Design review of the part built by this model. Coordinates are the model's own, in mm. A direction names the side the tool comes from. Coordinates: 2 decimals unless noted, no trailing zeros. Loops run counter-clockwise (first coordinate to the right, second up) from the corner with the lowest first, then second, coordinate; pieces in that order, holes last.
Autodesk Inventor part; units mm, degrees
ref_plane "Arbeitsebene2" through (0, 360, 0) normal (0, 1, 0) x (1, 0, 0)
ref_plane "YZ Plane" through (0, 0, 0) normal (1, 0, 0) x (0, 1, 0)
ref_plane "XZ Plane" through (0, 0, 0) normal (0, 1, 0) x (-1, 0, 0)
sketch "Skizze1" plane through (0, 0, 0) normal (0, 1, 0) x (-1, 0, 0)
  line L0 (599, 100) -> (-599, 100)
  line L1 (-599, 100) -> (-599, -100)
  line L2 (-599, -100) -> (599, -100)
  line L3 (599, -100) -> (599, 100)
  line L4 (838.6, 0) -> (-838.6, 0) construction
  line L5 (0, -140) -> (0, 140) construction
  point P0 (0, 0)
  dimension "d0" = 1198
  dimension "d1" = 200
extrude "Extrusion1" add sketch "Skizze1" along normal blind 420
shell "Wandung1" thickness 5 removed faces 1 at (199.6667, 0, -33.3333)
sketch "Skizze2" plane through (-599, 0, 100) normal (0, 0, 1) x (1, 0, 0)
  line L0 (0, 0) -> (1198, 0) construction
  line L1 (1198, 0) -> (1098, 0)
  line L2 (1098, 0) -> (1098, 130)
  line L3 (1098, 130) -> (1098, 360)
  point P0 (599, 0)
  dimension "d9" = 100
  dimension "d10" = 130
  dimension "d11" = 230
hole "Bohrung1" at (499, 360, 100) direction (0, 0, -1) diameter 30 depth 20 tip angle 118
ref_plane "Arbeitsebene1" through (0, 310.83, 0) normal (0, 1, 0) x (1, 0, 0)
sketch "Skizze3" plane through (0, 310.83, 0) normal (0, 1, 0) x (1, 0, 0)
  line L0 (599, 100) -> (-599, 100) construction
  line L1 (599, -100) -> (599, 100) construction
  line L2 (-599, -100) -> (599, -100) construction
  line L3 (-599, 100) -> (-599, -100) construction
  line L4 (599, -100) -> (499, -100)
  line L5 (499, -100) -> (511.5, -100)
  line L6 (499, -100) -> (486.5, -100)
  line L7 (-599, 100) -> (599, 100)
  line L8 (599, 100) -> (599, -100)
  line L9 (599, -100) -> (-599, -100)
  line L10 (-599, -100) -> (-599, 100)
  line L11 (599, 0) -> (86.8278, 0)
  line L12 (499, -100) -> (499, 0)
  line L13 (499, 0) -> (499, 100)
  line L14 (499, 0) -> (536.585, 0)
  line L15 (499, 0) -> (463.415, 0)
  line L16 (499, 0) -> (464.19, 0)
  line L17 (499, 0) -> (499, 36.585)
  line L18 (499, 36.585) -> (535.585, 36.585)
  line L19 (535.585, 36.585) -> (441.933, 36.585)
  line L20 (441.933, 36.585) -> (441.933, -36.585)
  line L21 (441.933, -36.585) -> (535.585, -36.585)
  line L22 (535.585, -36.585) -> (535.585, -71.395)
  line L23 (535.585, -71.395) -> (441.933, -71.395)
  line L24 (441.933, -71.395) -> (407.123, -71.395)
  line L25 (407.123, -71.395) -> (407.123, 36.585)
  line L26 (407.123, 36.585) -> (407.123, 71.395)
  line L27 (407.123, 71.395) -> (535.585, 71.395)
  line L28 (535.585, 71.395) -> (535.585, 36.585)
  point P0 (0, 0)
  dimension "d20" = 100
  dimension "d21" = 12.5
  dimension "d22" = 12.5
  dimension "d33" = 36.585
  dimension "d34" = 36.585
  dimension "d35" = 93.652
  dimension "d36" = 73.17
  dimension "d37" = 93.652
  dimension "d38" = 34.81
  dimension "d39" = 34.81
  dimension "d40" = 34.81
extrude "Extrusion2" add sketch "Skizze3" against normal blind 20
sketch "Skizze6" plane through (-599, 0, 100) normal (0, 0, 1) x (1, 0, 0)
  circle A0 centre (1098, 360) radius 15 construction
  line L0 (5, 310.83) -> (1193, 310.83) construction
  arc A1 (1113, 360) -> (1083, 360) centre (1098, 360) ccw
  line L1 (1083, 360) -> (1083, 310.83)
  line L2 (1113, 360) -> (1113, 310.83)
  circle A2 centre (1098, 360) radius 15
  point P0 (599, 0)
  dimension "d25" = 30
extrude "Extrusion3" add sketch "Skizze3" along normal blind 85 contours L23 L24 L25 L11 L20 L21 L12 | L12 L21 L22 L23 | L27 L28 L18 L13 | L13 L19 L20 L11 L25 L26 L27
ref_plane "Arbeitsebene2" through (0, 360, 0) normal (0, 1, 0) x (1, 0, 0)
sketch "Skizze7" plane through (0, 0, 0) normal (0, 0, 1) x (1, 0, 0)
  circle A0 centre (499, 360) radius 15 construction
  circle A1 centre (499, 360) radius 32
  circle A2 centre (499, 360) radius 32
  point P0 (0, 0)
  dimension "d44" = 64
extrude "Extrusion4" cut sketch "Skizze7" along normal mid plane 107.17
sketch "Skizze8" plane through (0, 420, 0) normal (0, 1, 0) x (1, 0, 0)
  line L0 (-599, 100) -> (599, 100)
  line L1 (599, 100) -> (599, -100)
  line L2 (599, -100) -> (-599, -100)
  line L3 (-599, -100) -> (-599, 100)
  point P0 (0, 0)
extrude "Extrusion5" cut sketch "Skizze8" against normal blind 5
hole "Bohrung2" at (499, 360, 100) direction (0, 0, -1) diameter 20 depth 500 tip angle 118
sketch "Skizze9" plane through (441.933, 310.83, -36.585) normal (1, 0, 0) x (0, 0, -1)
  line L0 (0, 0) -> (0, 85) construction
  line L1 (-73.17, 85) -> (0, 85) construction
  line L2 (-73.17, 0) -> (-73.17, 85) construction
  line L3 (-73.17, 85) -> (0, 85)
  line L4 (-73.17, 85) -> (-73.17, 0)
  line L5 (0, 0) -> (-73.17, 0)
  line L6 (-107.98, 0) -> (34.81, 0) construction
  line L7 (0, 0) -> (0, 85)
  line L8 (-36.585, 0) -> (-36.585, 49.17)
  circle A0 centre (-36.585, 49.17) radius 32
  circle A1 centre (-36.585, 49.17) radius 17.5
  point P0 (-36.585, -310.83)
  dimension "d56" = 49.17
  dimension "d58" = 64
  dimension "d61" = 35
extrude "Extrusion6" cut sketch "Skizze9" against normal blind 5 contours A1 | A0
extrude "Extrusion7" cut sketch "Skizze9" against normal blind 50 contours A1
sketch "Skizze10" plane through (0, 310.83, 0) normal (0, 1, 0) x (1, 0, 0)
  line L0 (-600.9138, 0) -> (-300.0038, 0)
  circle A0 centre (-300.0038, 0) radius 17.5
  line L1 (-300.0038, 0) -> (-206.3518, 0)
  line L2 (-262.3958, 0) -> (-262.3958, 70)
  line L3 (-262.3958, 70) -> (-232.3958, 70)
  line L4 (-232.3958, 70) -> (-232.3958, -70)
  line L5 (-232.3958, -70) -> (-262.3958, -70)
  line L6 (-262.3958, -70) -> (-262.3958, 0)
  line L7 (-300.0038, 0) -> (-263.4188, 0)
  line L8 (-300.0038, 0) -> (-262.3958, 0)
  point P0 (0, 0)
  dimension "d64" = 300.91
  dimension "d72" = 35
  dimension "d74" = 93.652
  dimension "d75" = 70
  dimension "d76" = 30
  dimension "d77" = 140
  dimension "d86" = 36.585
  dimension "d87" = 37.608
hole "Bohrung3" at (-300.0038, 310.83, 0) direction (0, -1, 0) diameter 64 depth 500 tip angle 118
extrude "Extrusion8" add sketch "Skizze10" along normal blind 104.17 contours L2 L3 L4 L1 | L1 L4 L5 L6
sketch "Skizze11" plane through (-262.3958, 310.83, -70) normal (-1, 0, 0) x (0, 0, 1)
  line L0 (-70, 49.17) -> (210, 49.17) construction
  circle A0 centre (70, 49.17) radius 17.5 construction
  circle A1 centre (70, 49.17) radius 32
  circle A2 centre (70, 49.17) radius 17.75
  point P0 (70, -310.83)
  dimension "d80" = 64
  dimension "d83" = 35.5
extrude "Extrusion9" cut sketch "Skizze11" against normal blind 12 contours A1 | A2
extrude "Extrusion10" cut sketch "Skizze11" against normal blind 40 contours A2
sketch "Skizze12" plane through (0, 310.83, 0) normal (0, 1, 0) x (1, 0, 0)
  circle A0 centre (-300.0038, 0) radius 32 construction
  circle A1 centre (-300.0038, 0) radius 40
  circle A2 centre (-300.0038, 0) radius 32
  point P0 (0, 0)
  dimension "d88" = 80
extrude "Extrusion11" add sketch "Skizze12" against normal blind 4
sketch "Skizze13" plane through (0, 0, 0) normal (0, -1, 0) x (1, 0, 0)
  circle A0 centre (-300.0038, 0) radius 32 construction
  circle A1 centre (-300.0038, 0) radius 12.5
  line L0 (-268.0493, -31.9545) -> (-331.9583, 31.9545) construction
  line L1 (-331.9583, -31.9545) -> (-268.0493, 31.9545) construction
  line L2 (-594, 95) -> (594, 95)
  line L3 (594, 95) -> (594, -95)
  line L4 (594, -95) -> (-594, -95)
  line L5 (-594, -95) -> (-594, 95)
  point P0 (0, 0)
  dimension "d101" = 25
extrude "Extrusion12" add sketch "Skizze13" against normal blind 10
sketch "Skizze14" plane through (599, 0, -100) normal (0, 0, -1) x (-1, 0, 0)
  circle A0 centre (100, 360) radius 10 construction
  circle A1 centre (100, 360) radius 15
  point P0 (599, 0)
  dimension "d104" = 30
hole "Bohrung4" at (499, 360, -100) direction (0, 0, 1) diameter 30 depth 20 tip angle 118
sketch "Skizze16" plane through (-232.3958, 310.83, 70) normal (1, 0, 0) x (0, 0, -1)
  circle A0 centre (70, 49.17) radius 17.75 construction
  circle A1 centre (70, 49.17) radius 23.5
  point P0 (70, -310.83)
  dimension "d112" = 47
extrude "Extrusion13" cut sketch "Skizze16" against normal blind 6.4
sketch "Skizze17" plane through (407.123, 310.83, 71.395) normal (-1, 0, 0) x (0, 0, 1)
  circle A0 centre (-71.395, 49.17) radius 17.5 construction
  circle A1 centre (-71.395, 49.17) radius 23.5
  point P0 (-71.395, -310.83)
  dimension "d115" = 47
extrude "Extrusion14" cut sketch "Skizze17" against normal blind 6.4
sketch "Skizze18" plane through (407.123, 310.83, 71.395) normal (0, 0, 1) x (1, 0, 0)
  circle A0 centre (91.877, 49.17) radius 10 construction
  circle A1 centre (91.877, 49.17) radius 16
  point P0 (-407.123, -310.83)
  dimension "d118" = 32
extrude "Extrusion15" cut sketch "Skizze18" against normal blind 7
sketch "Skizze19" plane through (535.585, 310.83, -71.395) normal (0, 0, -1) x (-1, 0, 0)
  circle A0 centre (36.585, 49.17) radius 16 construction
  circle A1 centre (36.585, 49.17) radius 16
  point P0 (535.585, -310.83)
  dimension "d121" = 32
extrude "Extrusion16" cut sketch "Skizze19" against normal blind 7
sketch "Skizze20" plane through (0, 310.83, 0) normal (0, 1, 0) x (1, 0, 0)
  circle A0 centre (-300.0038, 0) radius 32 construction
  circle A1 centre (-300.0038, 0) radius 40
  point P0 (0, 0)
  dimension "d124" = 80
extrude "Extrusion17" cut sketch "Skizze20" against normal blind 12
sketch "Skizze21" plane through (599, 0, -100) normal (0, 0, -1) x (-1, 0, 0)
  circle A0 centre (100, 360) radius 15 construction
  line L0 (1198, 415) -> (0, 415) construction
  line L1 (0, 0) -> (0, 415) construction
  line L2 (0, 0) -> (1198, 0) construction
  line L3 (1198, 0) -> (1198, 415) construction
  point P0 (599, 0)
sketch "Skizze22" plane through (0, 0, 0) normal (0, -1, 0) x (1, 0, 0)
  circle A0 centre (-356.8903, 42.7877) radius 5.0941 construction
  circle A1 centre (-298.864, 3.8435) radius 17.5 construction
  circle A2 centre (-298.864, 3.8435) radius 17.5 construction
  point P0 (0, 0)
  point P1 (-236.8903, 42.7877)
  point P2 (-236.8903, -47.2123)
  point P3 (-356.8903, -47.2123)
  point P4 (-236.8903, 42.7877)
  point P5 (-236.8903, -47.2123)
  point P6 (-356.8903, -47.2123)
hole "Bohrung5" at (-356.8903, 0, 42.7877) at (-236.8903, 0, 42.7877) at (-236.8903, 0, -47.2123) at (-356.8903, 0, -47.2123) direction (0, 1, 0) diameter 9.3762 depth 29.3 tip angle 118
sketch "Skizze23" plane through (0, 415, 0) normal (0, 1, 0) x (1, 0, 0)
  line L0 (-599, 100) -> (599, 100)
  line L1 (599, 100) -> (599, -100)
  line L2 (599, -100) -> (-599, -100)
  line L3 (-599, -100) -> (-599, 100)
  point P0 (0, 0)
extrude "Extrusion18" add sketch "Skizze23" along normal blind 10
properties part number "Mittelkonsole"
Q1. Take a section at A-A, the plane y = 271.5. Write out the cut boundary in (x, z).
Q2. For line 1 (Y direction, x = 438.45, z = 0); line 2 (Y direction, x = 208, z = -88); line 3 (X direction, y = 314.5, z = 47) (3 decimals), list the stretches that pass through material, from the lowest coordinate up.
Q3. The part is to be moulded in two halves that separate along Z. For faces 1 (the flat face through (-8, 148, 95)), 2 (the flat face through (-8, 425, -1)), 3 (the flat face through (436.933, 346, -14)), say which applies: pulls with the +Z half, pulls with the -Z half, needs draft (parallel to the pull), parting line crosses it, or undercut.
Q4. Machinability: for faces 4 (the flat face through (-8, 0, 1)), 5 (the cylindrical face through (529.522, 350.388, 44.966)), which of the approach directions +Z, -Z, +X, -X, +Y, -Y give a long, thin tool a straight path to every point of the face, cutting with its end or side? Answer none if there is none.
Q5. Take a section at B-B, the plane x = -203. Write out the cut boundary in (y, z), then the cut area to 4 significant figures.
Entries:
1. outline: (-599, -100) - (599, -100) - (599, 100) - (-599, 100) - close; hole (-594, -95) - (594, -95) - (594, 95) - (-594, 95) - close
2. line 1: y = 0 to 10, 290.83 to 328, 392 to 395.83, 415 to 425
2. line 2: y = 0 to 10, 290.83 to 310.83, 415 to 425
2. line 3: x = -599 to -594, -262.396 to -232.396, 407.123 to 535.585, 594 to 599
3. face 1: undercut
3. face 2: needs draft
3. face 3: undercut
4. face 4: +Z, -Z, +X, -X, -Y
4. face 5: none
5. outline: (0, -100) - (425, -100) - (425, 100) - (0, 100) - close; hole (10, -95) - (290.83, -95) - (290.83, 95) - (10, 95) - close; hole (310.83, -95) - (415, -95) - (415, 95) - (310.83, 95) - close
5. area: 11,850 mm2
